Could you check a few things on this drawing? It's one solid part, dimensions in mm from its lowest x, y, z. A direction names the side the tool comes from. Coordinates: 2 decimals unless noted, no trailing zeros. Write each loop counter-clockwise with the first axis right and the second up, starting at its lowest first coordinate (ties: lowest second). Pieces come first, ordered by that corner, then holes.
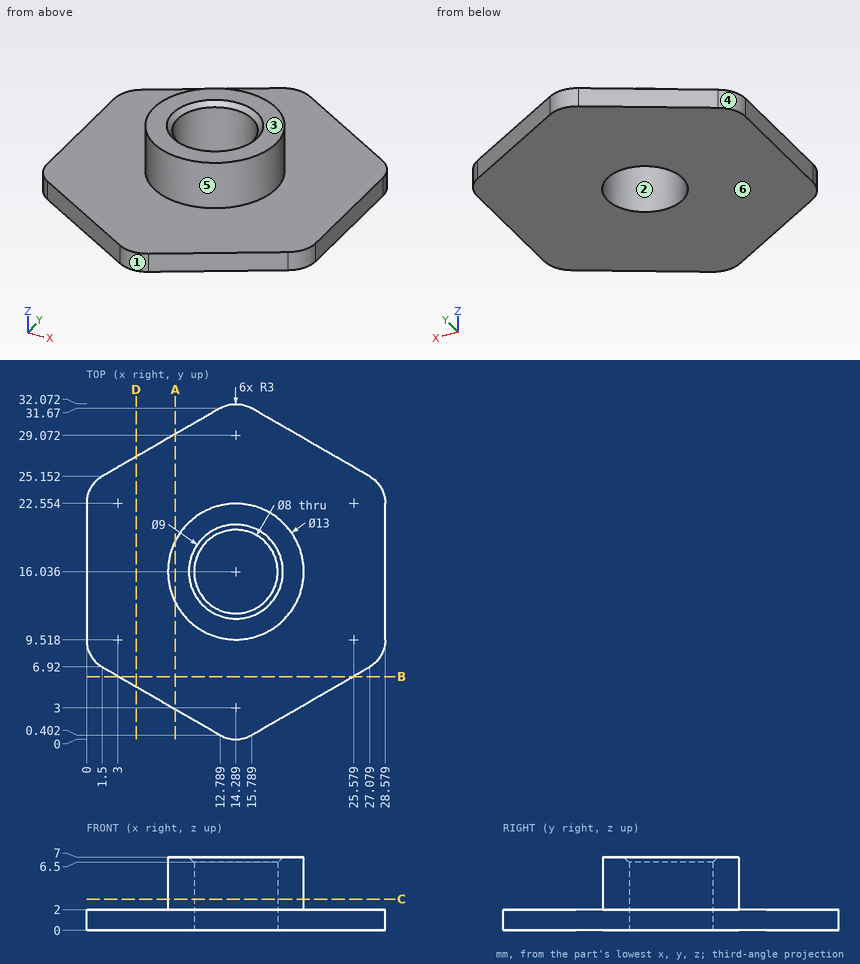
1) Imagine slicing it at D-D on x = 4.75. Please give me the cut outline in (y, z).
Values follow:
outline: (5.04, 0) - (27.03, 0) - (27.03, 2) - (5.04, 2) - close
2) On a 3-axis mill with a long thin cutter (end or side, diameter ignored), from which of +Z, -Z, +X, -X, +Y, -Y can I reach the whole of each face in a straight line? I mean the marked faces 5 and 6. Say none if no direction works.
Values follow:
face 5: +Z
face 6: -Z, +X, -X, +Y, -Y
3) Imagine slicing it at A-A on x = 8.5. Please give me the cut outline in (y, z).
Values follow:
outline: (2.88, 0) - (29.19, 0) - (29.19, 2) - (18.99, 2) - (18.99, 7) - (13.08, 7) - (13.08, 2) - (2.88, 2) - close
4) Imagine slicing it at C-C on z = 3. Please give me the cut outline in (x, y).
Values follow:
outline: circle Ø13 at (14.29, 16.04); hole circle Ø8 at (14.29, 16.04)
5) Will these pins go through, and if not, where does the flat tip stop? pin 1 (1 mm diameter, centred on x = 20, y = 25, fed in from -Z); pin 2 (1.5 mm diameter, centred on x = 24, z = 1, fed in from +Y); pin 3 (5 mm diameter, centred on x = 14.29, y = 16.04, fed in from +Z) (1 decimal).
Values follow:
pin 1: stops at z = 0
pin 2: stops at y = 27.36
pin 3: passes through
6) I need wall thicknesses on probe 1 along X at (y, z) = (16, 6.25); probe 2 along Z at (x, y) = (7, 22); probe 3 along X at (y, z) = (21, 5.5) (1 decimal). Which ranges of each line are inside material? Lowest first, please.
Values follow:
probe 1: x = 7.79 to 10.29, 18.29 to 20.79
probe 2: z = 0 to 2
probe 3: x = 10.1 to 18.5
7) Imagine slicing it at B-B on y = 6. Please give me the cut outline in (x, z) (1 decimal).
Values follow:
outline: (3.1, 0) - (25.5, 0) - (25.5, 2) - (3.1, 2) - close
8) We'd pull the mould along Y, two halves only. Please class the marked faces 1, 2, 3 and 4: pulls with the +Y half, pulls with the -Y half, needs draft (parallel to the pull), parting line crosses it, or undercut.
Values follow:
face 1: pulls with the -Y half
face 2: undercut
face 3: needs draft
face 4: pulls with the +Y half
